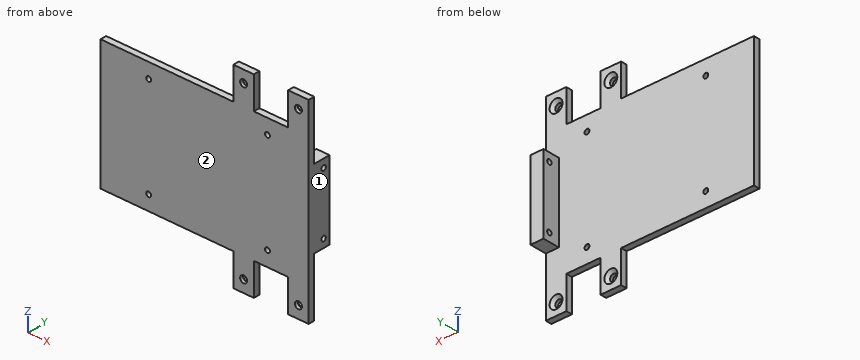
Autodesk Inventor part; units mm, degrees
ref_plane "YZ Plane" through (0, 0, 0) normal (1, 0, 0) x (0, 1, 0)
ref_plane "XZ Plane" through (0, 0, 0) normal (0, 1, 0) x (-1, 0, 0)
ref_plane "XY Plane" through (0, 0, 0) normal (0, 0, 1) x (1, 0, 0)
sketch "Sketch1" plane through (0, 0, 0) normal (0, 1, 0) x (-1, 0, 0)
  line L0 (-5, 47.5) -> (5, 47.5)
  line L1 (5, 47.5) -> (5, -47.5)
  line L2 (5, -47.5) -> (-5, -47.5)
  line L3 (-5, -47.5) -> (-5, 47.5)
  line L4 (-5, 47.5) -> (5, -47.5) construction
  line L5 (5, 47.5) -> (-5, -47.5) construction
  line L6 (-31.75, 31.75) -> (31.75, 31.75)
  line L7 (31.75, 31.75) -> (31.75, -31.75)
  line L8 (31.75, -31.75) -> (-31.75, -31.75)
  line L9 (-31.75, -31.75) -> (-31.75, 31.75)
  line L10 (-31.75, 31.75) -> (31.75, -31.75) construction
  line L11 (31.75, 31.75) -> (-31.75, -31.75) construction
  line L12 (31.75, 31.75) -> (69.85, 31.75)
  line L13 (69.85, 31.75) -> (69.85, -31.75)
  line L14 (69.85, -31.75) -> (31.75, -31.75)
  line L15 (31.75, -31.75) -> (31.75, 31.75)
  line L16 (-31.75, 0) -> (-26.7462, 0)
  line L17 (-21.7424, 47.6123) -> (-31.75, 47.6123)
  line L18 (-31.75, 47.6123) -> (-31.75, -47.6123)
  line L19 (-31.75, -47.6123) -> (-21.7424, -47.6123)
  line L20 (-21.7424, -47.6123) -> (-21.7424, 47.6123)
  line L21 (-21.7424, 47.6123) -> (-31.75, -47.6123) construction
  line L22 (-31.75, 47.6123) -> (-21.7424, -47.6123) construction
  point P0 (0, 0)
  point P1 (-5, -31.75)
  point P2 (-5, 31.75)
  point P3 (31.75, 31.75)
  point P4 (5, 31.75)
  point P5 (5, -31.75)
  point P6 (-21.7424, -31.75)
  point P7 (-21.7424, 31.75)
  dimension "d0" = 10
  dimension "d1" = 95
  dimension "d13" = 63.5
  dimension "d14" = 63.5
  dimension "d15" = 38.1
  dimension "d47" = 5.0038
  dimension "d48" = 95.2246
extrude "Extrusion1" add sketch "Sketch1" along normal blind 3
sketch "Sketch2" plane through (0, 3, 0) normal (0, 1, 0) x (1, 0, 0)
  line L0 (0, 0) -> (0, 41.65)
  line L1 (0, 0) -> (0, -41.65)
  line L2 (21.7424, -47.6123) -> (31.75, -47.6123)
  line L3 (26.7462, -47.6123) -> (26.7462, 0)
  line L4 (26.7462, 0) -> (26.7462, 41.656)
  line L5 (26.7462, 0) -> (26.7462, -41.656)
  dimension "d4" = 41.65
  dimension "d5" = 41.65
  dimension "d49" = 41.656
  dimension "d50" = 41.656
hole "Hole1" at (0, 3, 41.65) at (0, 3, -41.65) at (26.7462, 3, 41.656) at (26.7462, 3, -41.656) direction (0, -1, 0) diameter 3.4036 end through all countersink diameter 6.2992 countersink angle 90
sketch "Sketch3" plane through (0, 3, 0) normal (0, 1, 0) x (1, 0, 0)
  line L0 (31.75, -31.75) -> (31.75, 31.75)
  line L1 (31.75, 0) -> (28.575, 0)
  line L2 (25.4, -19.05) -> (31.75, -19.05)
  line L3 (31.75, -19.05) -> (31.75, 19.05)
  line L4 (31.75, 19.05) -> (25.4, 19.05)
  line L5 (25.4, 19.05) -> (25.4, -19.05)
  line L6 (25.4, -19.05) -> (31.75, 19.05) construction
  line L7 (31.75, -19.05) -> (25.4, 19.05) construction
  point P0 (0, 0)
  dimension "d16" = 3.175
  dimension "d17" = 38.1
extrude "Extrusion2" add sketch "Sketch3" along normal blind 8.255
sketch "Sketch4" plane through (31.75, 0, 31.75) normal (1, 0, 0) x (0, 0, -1)
  line L0 (12.7, 11.255) -> (50.8, 11.255)
  line L1 (31.75, 11.255) -> (31.75, 8.08)
  line L2 (31.75, 8.08) -> (46.75, 8.08)
  line L3 (46.75, 8.08) -> (16.75, 8.08)
  point P0 (31.75, 0)
  dimension "d20" = 3.175
  dimension "d21" = 15
  dimension "d22" = 30
hole "Hole2" at (31.75, 8.08, 15) at (31.75, 8.08, -15) direction (-1, 0, 0) diameter 2.3876 end through all
sketch "Sketch5" plane through (0, 3, 0) normal (0, 1, 0) x (1, 0, 0)
  line L0 (-69.85, 31.75) -> (-69.85, -31.75)
  line L1 (-69.85, 0) -> (-69.85, 24.5)
  line L2 (-69.85, 24.5) -> (-69.85, -24.5)
  line L3 (-69.85, -24.5) -> (15.15, -24.5)
  line L4 (15.15, -24.5) -> (-69.85, -24.5)
  line L5 (-69.85, -24.5) -> (-69.85, 24.5)
  line L6 (-69.85, 24.5) -> (15.15, 24.5)
  line L7 (15.15, 24.5) -> (15.15, -24.5)
  line L8 (15.15, -24.5) -> (11.65, -24.5)
  line L9 (11.65, -24.5) -> (11.65, -21)
  line L10 (11.65, -21) -> (15.15, -21)
  line L11 (15.15, -21) -> (15.15, -24.5)
  line L12 (15.15, 24.5) -> (11.65, 24.5)
  line L13 (11.65, 24.5) -> (11.65, 21)
  line L14 (11.65, 21) -> (15.15, 21)
  line L15 (15.15, 21) -> (15.15, 24.5)
  line L16 (11.65, -21) -> (-46.35, -21)
  line L17 (11.65, -21) -> (69.65, -21) construction
  line L18 (11.65, 21) -> (-46.35, 21)
  line L19 (-46.35, 21) -> (-46.35, 24.5)
  line L20 (-46.35, -21) -> (-46.35, -24.5)
  point P0 (0, 0)
  dimension "d30" = 24.5
  dimension "d31" = 49
  dimension "d32" = 85
  dimension "d33" = 3.5
  dimension "d34" = 3.5
  dimension "d35" = 3.5
  dimension "d36" = 3.5
  dimension "d37" = 58
  dimension "d38" = 180
  dimension "d39" = 58
hole "Hole3" at (11.65, 3, 24.5) at (11.65, 3, -24.5) at (-46.35, 3, -24.5) at (-46.35, 3, 24.5) direction (0, -1, 0) diameter 2.3876 end through all
properties part number "OT2-ridingcam-r1"
Design review of the part built by this model. Coordinates are the model's own, in mm. Face numbers are marked on the shaded views. Coordinates: 2 decimals unless noted, no trailing zeros. Loops run counter-clockwise (first coordinate to the right, second up) from the corner with the lowest first, then second, coordinate; pieces in that order, holes last. Notation, with made-up numbers: (-27.5, 79.5) -> (-10.5, 79.5) arc R27 ccw to (-10.5, 100.5) -> close; hole circle Ø8 at (-39, 77). An arc over 180 degrees is marked (long way). Use a Markdown table: item, result. Add a question column.
Item 1: We need section A-A, the plane z = 24.5. Write out the cut boundary in (x, y), and give its area (3 significant figures).
Item 2: The part is to be moulded in two halves that separate along Y. For the marked faces 1 and 2, say which applies: +Y half, -Y half, draft (parallel to the pull), parting line (faces both ways), or undercut.
Item 3: We need section D-D, the plane z = -5. Write out the cut boundary in (x, y) (3 decimals).
Item 4: Clearance check with flat-ended pins moving along their axes: P1, Ø6, axis at x = -12, y = 1.5, coming from the -Z side; P2, Ø4, axis at x = 26.75, z = 41.66, coming from the +Y side; P3, Ø6, axis at x = -25, y = 2.5, coming from the +Z side. State where each tip first meets the part, or that it passes through.
Item 5: We need section B-B, the plane x = 11.65. Write out the cut boundary in (y, z), and give its area (3 significant figures).
Item 6: We need section C-C, the plane z = -15. Write out the cut boundary in (x, y) (3 decimals).
Item 7: Wall thickness on L1, parallel to Z at x = 0, y = 0.65; L2, parallel to X at y = 1.95, z = 24.5; L3, parallel to Y at x = 26.75, z = -15 (3 decimals): over which ranges is each line inside the solid? List them lowest first. Write a range as from..to.
Numbers:
| question | item | result |
|---|---|---|
| 1 | outline | (-69.85, 0) -> (-47.54, 0) -> (-47.54, 3) -> (-69.85, 3) -> close; (-45.16, 0) -> (10.46, 0) -> (10.46, 3) -> (-45.16, 3) -> close; (12.84, 0) -> (31.75, 0) -> (31.75, 3) -> (12.84, 3) -> close |
| 1 | area | 290 mm^2 |
| 2 | face 1 | draft |
| 2 | face 2 | -Y half |
| 3 | outline | (-69.85, 0) -> (31.75, 0) -> (31.75, 11.255) -> (25.4, 11.255) -> (25.4, 3) -> (-69.85, 3) -> close |
| 4 | P1 | stops at z = -31.75 |
| 4 | P2 | stops at y = 1.86 |
| 4 | P3 | stops at z = 31.75 |
| 5 | outline | (0, -31.75) -> (3, -31.75) -> (3, -25.69) -> (0, -25.69) -> close; (0, -23.31) -> (3, -23.31) -> (3, 23.31) -> (0, 23.31) -> close; (0, 25.69) -> (3, 25.69) -> (3, 31.75) -> (0, 31.75) -> close |
| 5 | area | 176 mm^2 |
| 6 | outline | (-69.85, 0) -> (31.75, 0) -> (31.75, 6.886) -> (25.4, 6.886) -> (25.4, 3) -> (-69.85, 3) -> close; (25.4, 9.274) -> (31.75, 9.274) -> (31.75, 11.255) -> (25.4, 11.255) -> close |
| 7 | L1 | z = -47.5..-43.35, -39.95..39.95, 43.35..47.5 |
| 7 | L2 | x = -69.85..-47.54, -45.16..10.46, 12.84..31.75 |
| 7 | L3 | y = 0..6.886, 9.274..11.255 |
